```python
from build123d import *

# Parameters (mm, degrees)
SKETCH2_W           = 13
SKETCH2_H           = 8
SKETCH1_W           = 14
SKETCH1_H           = 8.95
SKETCH3_W           = 14
SKETCH3_H           = 8.95
BOSS_EXTRUDE1_DEPTH = 1
SKETCH4_W           = 16
SKETCH4_H           = 10.95
BOSS_EXTRUDE2_DEPTH = 1
FILLET1_R           = 2
CHAMFER1_SIZE       = 0.5
FILLET2_R           = 0.5


with BuildPart() as part:
    # Sketch2 → Loft1 section 0
    with BuildSketch(Plane.XY.offset(2)):
        Rectangle(SKETCH2_W, SKETCH2_H)
    # Sketch1 → Loft1 section 1
    with BuildSketch(Plane.XY):
        Rectangle(SKETCH1_W, SKETCH1_H)
    loft()

    # Sketch3 → Boss-Extrude1 (add)
    with BuildSketch(Plane(origin=(0, 0, 0), x_dir=(-1, 0, 0), z_dir=(0, 0, -1))):
        Rectangle(SKETCH3_W, SKETCH3_H)
    extrude(amount=BOSS_EXTRUDE1_DEPTH)

    # Sketch4 → Boss-Extrude2 (add)
    with BuildSketch(Plane(origin=(0, 0, -1), x_dir=(-1, 0, 0), z_dir=(0, 0, -1))):
        Rectangle(SKETCH4_W, SKETCH4_H)
    extrude(amount=BOSS_EXTRUDE2_DEPTH)

    # Fillet1
    fillet1_edges = [part.edges().sort_by_distance(p)[0] for p in [
        (-8, -5.475, -1.5),
        (-8, 5.475, -1.5),
        (8, 5.475, -1.5),
        (8, -5.475, -1.5),
    ]]
    fillet(fillet1_edges, radius=FILLET1_R)

    # Chamfer1
    chamfer1_edges = [part.edges().sort_by_distance(p)[0] for p in [
        (-8, 0, -2),
        (0, -5.475, -2),
        (0, 5.475, -2),
        (8, 0, -2),
        (7.414213562, 4.889213562, -2),
        (7.414213562, -4.889213562, -2),
        (-7.414213562, 4.889213562, -2),
        (-7.414213562, -4.889213562, -2),
    ]]
    chamfer(chamfer1_edges, length=CHAMFER1_SIZE)

    # Fillet2
    fillet2_edges = [part.edges().sort_by_distance(p)[0] for p in [
        (-7, -4.475, -0.5),
        (-7, 4.475, -0.5),
        (7, -4.475, -0.5),
        (7, 4.475, -0.5),
    ]]
    fillet(fillet2_edges, radius=FILLET2_R)


solid = part.part
```
Geometry check sheet. Reference: the model listing, model coordinates, mm. A direction names the side the tool comes from. Coordinates: 2 decimals unless noted, no trailing zeros.
Item 1: Tool access check on faces 1 (the flat face through (0.1, -4.475, -0.5)), 2 (the flat face through (-7, -0.1, -0.5)), 3 (the flat face through (0, 5, -1)), 4 (the flat face through (7, -0.1, -0.5)). Record the directions out of +Z, -Z, +X, -X, +Y, -Y that give a thin tool (end or side, any length) a straight path to the whole face; none if there is none.
Item 2: Mould release check, pull along X, two halves, no side actions. Record for faces 5 (the cylindrical face through (7.43, -4.874, -1.254)), 6 (the conical face through (-7.149, -4.649, -1.858)), 7 (the flat face through (0.1, 4.475, -0.5)): released by +X, released by -X, zero draft, split by the parting line, or undercut.
Item 3: Scan lines: line 1 along Y through (x, z) = (4.75, 0.6); line 2 along X through (y, z) = (0.5, -0.4); line 3 along Z through (x, y) = (6, 4.75). Record each from-to range of solid material in increasing order.
Item 4: Depth check by flat-ended pin: pin 1 (1.5 mm diameter, centred on x = 4, z = 1, fed in from -Y); pin 2 (0.5 mm diameter, centred on y = 0, z = -0.5, fed in from -X); pin 3 (0.8 mm diameter, centred on y = -2, z = -0.5, fed in from +X). Enter the tip coordinate at first touch or a pass-through.
Check sheet entries:
1. face 1: +Z, +X, -X, -Y
1. face 2: +Z, -X, +Y, -Y
1. face 3: +Z
1. face 4: +Z, +X, +Y, -Y
2. face 5: released by +X
2. face 6: released by -X
2. face 7: zero draft
3. line 1: y = -4.33 to 4.33
3. line 2: x = -7 to 7
3. line 3: z = -2 to -1
4. pin 1: stops at y = -4.42
4. pin 2: stops at x = -7
4. pin 3: stops at x = 7
